from build123d import *

# Parameters (mm, degrees)
F0_W     = 160
F0_H     = 6
F1_DEPTH = 6
F2_R     = 2.99999
F4_D     = 4


# Not quite as in the source:
# - a fillet or chamfer is up to 0.001 mm smaller than in the source, because OpenCascade refuses the exact size


with BuildPart() as f1:
    # F0 (on Top) → F1 (new body)
    with BuildSketch(Plane.XY):
        with Locations((0.9389727563, 14.3314650139)):
            Rectangle(F0_W, F0_H)
    extrude(amount=F1_DEPTH)

    # F2 (radius 3 in the source; OpenCascade refuses exactly that, so slightly less here)
    f2_edges = [f1.edges().sort_by_distance(p)[0] for p in [
        (0.938973, 17.331465, 6),
        (0.938973, 11.331465, 6),
        (0.938973, 17.331465, 0),
        (0.938973, 11.331465, 0),
    ]]
    fillet(f2_edges, radius=F2_R)

    # F4 (through all)
    with Locations(Plane.YZ.offset(80.9389727563)):
        with Locations((14.3314650139, 3)):
            Hole(F4_D / 2)


solid = f1.part
Part model, mm, in its own coordinate system. Round coordinates to 2 decimals unless told otherwise and drop trailing zeros. Put each result on its own line as item: value.
Q1. Wall check: line 1 (Z direction, x = 71.5, y = 14.5); line 2 (Y direction, x = 45, z = 2.85); line 3 (Y direction, x = -41, z = 3.55). Give the ranges that are in metal, low to high. Write a range as [from, to].
From the geometry:
line 1: z = [0, 1.01], [4.99, 6]
line 2: y = [11.34, 12.34], [16.33, 17.33]
line 3: y = [11.38, 12.41], [16.25, 17.28]
Q2. Pin check, flat tips, straight feed: pin 1 Ø3 at (x, y) = (26, 12.5) entering from +Z; pin 2 Ø1.5 at (x, y) = (-21, 15.5) entering from -Z; pin 3 Ø2.5 at (y, z) = (14.33, 3) entering from +X; pin 4 Ø3 at (x, y) = (-41.5, 12) entering from +Z. Stop position of each tip, or through.
From the geometry:
pin 1: stops at z = 5.98
pin 2: stops at z = 0.03
pin 3: passes through
pin 4: stops at z = 5.88
Q3. Pull direction Z, two halves, no side cores. Call faces 1 (the face through (-0.181, 15.919, 1.783)), 2 (the face through (2.06, 12.19, 0.9)), 3 (the face through (80.939, 12, 3)): pulls with the +Z half, pulls with the -Z half, needs draft (parallel to the pull), parting line crosses it, or undercut.
From the geometry:
face 1: undercut
face 2: pulls with the -Z half
face 3: needs draft
